from build123d import *

# Parameters (mm, degrees)
F0_W     = 22
F0_H     = 24
F3_DEPTH = 4
F4_D     = 13.4
F5_D     = 3.6


with BuildPart() as f3:
    # F0 (on Top) → F3 (new body)
    with BuildSketch(Plane.XY):
        Rectangle(F0_W, F0_H)
    extrude(amount=F3_DEPTH)

    # F4 (through all)
    with Locations(Plane(origin=(0, 0, 0), x_dir=(1, 0, 0), z_dir=(0, 0, -1))):
        with Locations((0, 0)):
            Hole(F4_D / 2)

    # F5 (through all)
    with Locations(Plane(origin=(0, 0, 0), x_dir=(1, 0, 0), z_dir=(0, 0, -1))):
        with Locations((0, 10)):
            Hole(F5_D / 2)


solid = f3.part
Can you work these out from the model? Positions are in its coordinate system, mm. Give positions to 0.01 mm unless a question says otherwise; leave off trailing zeros. Order: outer loops, then holes, each group sorted by start corner. A loop starts at its lowest first (then second) coordinate and runs counter-clockwise, first axis right, second up. Notation, with made-up numbers: M 27.25,13 L 47.25,13 A8 ccw 47.25,19 Z; hole C 5.5,65.5 d6. An arc over 180 degrees is marked long. Use one line per item in the form item = value.
Item 1: Thinking about a two-plate mould opening in Y: for faces 1 (the flat face through (0, 12, 2)), 2 (the cylindrical face through (6.694, -0.295, 2.028)), 3 (the flat face through (11, 0, 2)), which applies, pulls with the +Y half, pulls with the -Y half, needs draft (parallel to the pull), parting line crosses it, or undercut?
Values follow:
face_1 = pulls with the +Y half
face_2 = undercut
face_3 = needs draft
Item 2: If I drill on line 1 along Y through (x, z) = (0, 1.65); line 2 along X through (y, z) = (0.25, 1.15); line 3 along Y through (x, z) = (1, 1.95), over which ranges is the centre line in solid material (lowest first)? Write a range as [from, to].
Values follow:
line_1 = [-12, -11.8], [-8.2, -6.7], [6.7, 12]
line_2 = [-11, -6.7], [6.7, 11]
line_3 = [-12, -11.5], [-8.5, -6.62], [6.62, 12]
Item 3: If we section it at C-C, the plane x = -4.5: Write out the boundary of the cut face in (y, z).
Values follow:
outline = M -12,0 L -4.96,0 L -4.96,4 L -12,4 Z; M 4.96,0 L 12,0 L 12,4 L 4.96,4 Z
Item 4: If we section it at D-D, the plane z = 2.6: Write out the boundary of the cut face in (x, y), and give its area (3 significant figures).
Values follow:
outline = M -11,-12 L 11,-12 L 11,12 L -11,12 Z; hole C 0,0 d13.4; hole C 0,-10 d3.6
area = 377 mm^2
Item 5: If we section it at A-A, the plane y = -10: Write out the boundary of the cut face in (x, z), and give its area (3 significant figures).
Values follow:
outline = M -11,0 L -1.8,0 L -1.8,4 L -11,4 Z; M 1.8,0 L 11,0 L 11,4 L 1.8,4 Z
area = 73.6 mm^2
Item 6: If we section it at B-B, the plane x = 0: Write out the boundary of the cut face in (y, z), and give its area (3 significant figures).
Values follow:
outline = M -12,0 L -11.8,0 L -11.8,4 L -12,4 Z; M -8.2,0 L -6.7,0 L -6.7,4 L -8.2,4 Z; M 6.7,0 L 12,0 L 12,4 L 6.7,4 Z
area = 28.0 mm^2
Item 7: Will this pin go through, and if not, where does the flat tip stop? pin 1 Ø3 at (x, y) = (0, -10) entering from +Z.
Values follow:
pin_1 = through
